```python
from build123d import *

# Parameters (mm, degrees)
BOSS_EXTRUDE1_DEPTH = 1.9


with BuildPart() as part:
    # Sketch1 → Boss-Extrude1 (new, symmetric)
    with BuildSketch(Plane(origin=(0, 0, 0), x_dir=(0, 0, -1), z_dir=(1, 0, 0))):
        with BuildLine():
            Line((-84.195498156, -182.4), (-80, -182.4))
            Line((-80, -182.4), (20, -182.4))
            Line((20, -182.4), (20, -167.4))
            Line((20, -167.4), (-80, -167.4))
            Line((-80, -167.4), (-84.195498156, -167.4))
            ThreePointArc((-84.195498156, -167.4), (-90.623374253, -165.060444431), (-94.043575686, -159.136481777))
            Line((-94.043575686, -159.136481777), (-116.478138504, -31.903753538))
            Line((-116.478138504, -31.903753538), (-131.250254799, -34.508476203))
            Line((-131.250254799, -34.508476203), (-108.815691981, -161.741204442))
            ThreePointArc((-108.815691981, -161.741204442), (-100.265188398, -176.551111078), (-84.195498156, -182.4))
        make_face()
    extrude(amount=BOSS_EXTRUDE1_DEPTH, both=True)


solid = part.part
```
Source: CAD feature listing. Evaluate the final solid. Frame: model axes, mm. A direction names the side the tool comes from. Round coordinates to 2 decimals unless told otherwise and drop trailing zeros. Loops run counter-clockwise (first coordinate to the right, second up) from the corner with the lowest first, then second, coordinate; pieces in that order, holes last.
1. Section query B-B on z = 33.5. Output: boundary loops of the cut face in (x, y).
2. Section query A-A on x = 0.55. Output: boundary loops of the cut face in (y, z), and give its area (3 significant figures).
3. Access query for faces 1 (the flat face through (0, -167.4, 31)), 2 (the cylindrical face through (0.027, -176.393, 100.452)). Directions: +Z, -Z, +X, -X, +Y, -Y. A direction counts if a zero-diameter tool reaches every point of the face in a straight line with its end or side. Return the directions, or none.
4. Contact query for flat-ended pins moving along their axis: pin 1 (1.5 mm diameter, centred on x = 1, z = 58, fed in from +Y); pin 2 (1.5 mm diameter, centred on x = -0.5, y = -57, fed in from +Z). Output: stop coordinate, or through.
5. Section query C-C on y = -164. Output: boundary loops of the cut face in (x, z), and give its area (3 significant figures).
6. Ray query, L1, parallel to Y at x = 1.75, z = 41; L2, parallel to Z at x = -0.6, y = -90.5; L3, parallel to Z at x = 0.55, y = -173.5. Return the intervals inside material, ascending.
Answers below:
1. outline: (-1.9, -182.4) - (1.9, -182.4) - (1.9, -167.4) - (-1.9, -167.4) - close
2. outline: (-182.4, -20) - (-167.4, -20) - (-167.4, 84.2) arc R10 cw to (-159.14, 94.04) - (-31.9, 116.48) - (-34.51, 131.25) - (-161.74, 108.82) arc R25 ccw to (-182.4, 84.2) - close
2. area: 3,870 mm2
3. face 1: -Z, +X, -X, +Y
3. face 2: +Z, +X, -X, -Y
4. pin 1: stops at y = -167.4
4. pin 2: stops at z = 127.42
5. outline: (-1.9, 91.71) - (1.9, 91.71) - (1.9, 108.31) - (-1.9, 108.31) - close
5. area: 63.1 mm2
6. L1: y = -182.4 to -167.4
6. L2: z = 106.15 to 121.38
6. L3: z = -20 to 103.32
